CAD build for the part. Positions are in the model's coordinates, mm. Face numbers are marked on the shaded views. A direction names the side the tool comes from. Round coordinates to 2 decimals unless told otherwise and drop trailing zeros. Order: outer loops, then holes, each group sorted by start corner. A loop starts at its lowest first (then second) coordinate and runs counter-clockwise, first axis right, second up. Notation, with made-up numbers: M 35,63.25 L 80,63.25 A26 ccw 80,88.25 Z; hole C 30.25,15 d1. An arc over 180 degrees is marked long. Put each result on its own line as item: value.
```python
from build123d import *

# Parameters (mm, degrees)
SKETCH1_W                    = 52.6
SKETCH1_H                    = 21
BASE_FLANGE1_DEPTH           = 2
EDGE_FLANGE1_STRIP_W         = 9
EDGE_FLANGE1_STRIP_H         = 2
EDGE_FLANGE1_STRIP_CUT_DEPTH = 21
EDGE_FLANGE1_DEPTH           = 21
EDGE_FLANGE2_STRIP_W         = 9
EDGE_FLANGE2_STRIP_H         = 2
EDGE_FLANGE2_STRIP_CUT_DEPTH = 21
EDGE_FLANGE2_DEPTH           = 21
EDGE_FLANGE3_STRIP_W         = 9
EDGE_FLANGE3_STRIP_H         = 2
EDGE_FLANGE3_STRIP_CUT_DEPTH = 21
EDGE_FLANGE3_DEPTH           = 21
SKETCH15_W                   = 3.4
SKETCH15_H                   = 7
CUT_EXTRUDE1_DEPTH           = 10
SKETCH16_R                   = 1.25
CUT_EXTRUDE2_DEPTH           = 2
SKETCH18_W                   = 5.7
SKETCH18_H                   = 7
CUT_EXTRUDE3_DEPTH           = 39.376425055
SKETCH19_R                   = 2.95
CUT_EXTRUDE4_DEPTH           = 2
SKETCH20_R                   = 1.25
CUT_EXTRUDE5_DEPTH           = 2
SKETCH21_R                   = 8.25
CUT_EXTRUDE6_DEPTH           = 2
MOVE_FACE1_BY                = 0.8


# Sheet-metal steps are written as plain solids
with BuildPart() as part:
    # Sketch1 → Base-Flange1 (new body)
    with BuildSketch(Plane(origin=(0, 0, 0), x_dir=(1, 0, 0), z_dir=(0, 1, 0))):
        Rectangle(SKETCH1_W, SKETCH1_H)
    extrude(amount=-BASE_FLANGE1_DEPTH)

    # Edge-Flange1 strip (across the edge) → Edge-Flange1 strip cut (cut)
    with BuildSketch(Plane(origin=(-26.3, 0, -10.5), x_dir=(1, 0, 0), z_dir=(0, 0, 1))):
        with Locations((-2, -1)):
            Rectangle(EDGE_FLANGE1_STRIP_W, EDGE_FLANGE1_STRIP_H)
    extrude(amount=EDGE_FLANGE1_STRIP_CUT_DEPTH, mode=Mode.SUBTRACT)

    # Edge-Flange1 section (across the edge) → Edge-Flange1 (add)
    with BuildSketch(Plane(origin=(-26.3, 0, -10.5), x_dir=(1, 0, 0), z_dir=(0, 0, 1))):
        with BuildLine():
            Line((0, 0.5), (0, 23.9))
            Line((0, 23.9), (2, 23.9))
            Line((2, 23.9), (2, 0.5))
            ThreePointArc((2, 0.5), (2.146446609, 0.146446609), (2.5, 0))
            Line((2.5, 0), (2.5, -2))
            ThreePointArc((2.5, -2), (0.732233047, -1.267766953), (0, 0.5))
        make_face()
    extrude(amount=EDGE_FLANGE1_DEPTH)

    # Edge-Flange2 strip (across the edge) → Edge-Flange2 strip cut (cut)
    with BuildSketch(Plane(origin=(-24.3, 23.9, -10.5), x_dir=(0, -1, 0), z_dir=(0, 0, 1))):
        with Locations((-2, -1)):
            Rectangle(EDGE_FLANGE2_STRIP_W, EDGE_FLANGE2_STRIP_H)
    extrude(amount=EDGE_FLANGE2_STRIP_CUT_DEPTH, mode=Mode.SUBTRACT)

    # Edge-Flange2 section (across the edge) → Edge-Flange2 (add)
    with BuildSketch(Plane(origin=(-24.3, 23.9, -10.5), x_dir=(0, -1, 0), z_dir=(0, 0, 1))):
        with BuildLine():
            Line((0, 0.5), (0, 34.8))
            Line((0, 34.8), (2, 34.8))
            Line((2, 34.8), (2, 0.5))
            ThreePointArc((2, 0.5), (2.146446609, 0.146446609), (2.5, 0))
            Line((2.5, 0), (2.5, -2))
            ThreePointArc((2.5, -2), (0.732233047, -1.267766953), (0, 0.5))
        make_face()
    extrude(amount=EDGE_FLANGE2_DEPTH)

    # Edge-Flange3 strip (across the edge) → Edge-Flange3 strip cut (cut)
    with BuildSketch(Plane(origin=(26.3, 0, 10.5), x_dir=(-1, 0, 0), z_dir=(0, 0, -1))):
        with Locations((-2, -1)):
            Rectangle(EDGE_FLANGE3_STRIP_W, EDGE_FLANGE3_STRIP_H)
    extrude(amount=EDGE_FLANGE3_STRIP_CUT_DEPTH, mode=Mode.SUBTRACT)

    # Edge-Flange3 section (across the edge) → Edge-Flange3 (add)
    with BuildSketch(Plane(origin=(26.3, 0, 10.5), x_dir=(-1, 0, 0), z_dir=(0, 0, -1))):
        with BuildLine():
            Line((0, 0.5), (0, 21.6))
            Line((0, 21.6), (2, 21.6))
            Line((2, 21.6), (2, 0.5))
            ThreePointArc((2, 0.5), (2.146446609, 0.146446609), (2.5, 0))
            Line((2.5, 0), (2.5, -2))
            ThreePointArc((2.5, -2), (0.732233047, -1.267766953), (0, 0.5))
        make_face()
    extrude(amount=EDGE_FLANGE3_DEPTH)

    # Sketch15 → Cut-Extrude1 (cut)
    with BuildSketch(Plane(origin=(0, 23.9, 0), x_dir=(1, 0, 0), z_dir=(0, 1, 0))):
        with Locations((8.8, 0)):
            Rectangle(SKETCH15_W, SKETCH15_H)
    extrude(amount=-CUT_EXTRUDE1_DEPTH, mode=Mode.SUBTRACT)

    # Sketch16 → Cut-Extrude2 (cut)
    with BuildSketch(Plane(origin=(0, 23.9, 0), x_dir=(1, 0, 0), z_dir=(0, 1, 0))):
        with Locations(Location((4.1, 7.8, 0), (0, 0, 180))):
            Circle(SKETCH16_R)
        with Locations(Location((-15.9, -7.3, 0), (0, 0, 180))):
            Circle(SKETCH16_R)
    extrude(amount=-CUT_EXTRUDE2_DEPTH, mode=Mode.SUBTRACT)

    # Sketch18 → Cut-Extrude3 (cut, through all)
    with BuildSketch(Plane(origin=(0, 23.9, 0), x_dir=(1, 0, 0), z_dir=(0, 1, 0))):
        with Locations((9.95, 0)):
            Rectangle(SKETCH18_W, SKETCH18_H)
    extrude(amount=-CUT_EXTRUDE3_DEPTH, mode=Mode.SUBTRACT)

    # Sketch19 → Cut-Extrude4 (cut)
    with BuildSketch(Plane.ZY.offset(26.3)):
        with Locations(Location((0, 10.95, 0), (0, 0, 270))):
            Circle(SKETCH19_R)
    extrude(amount=-CUT_EXTRUDE4_DEPTH, mode=Mode.SUBTRACT)

    # Sketch20 → Cut-Extrude5 (cut)
    with BuildSketch(Plane.XZ.offset(2)):
        with Locations(Location((-16.55, 7.1, 0), (0, 0, 270))):
            Circle(SKETCH20_R)
        with Locations(Location((3.05, 7.1, 0), (0, 0, 270))):
            Circle(SKETCH20_R)
        with Locations(Location((18.05, 7.1, 0), (0, 0, 270))):
            Circle(SKETCH20_R)
        with Locations(Location((-16.55, -7.1, 0), (0, 0, 270))):
            Circle(SKETCH20_R)
        with Locations(Location((3.05, -7.1, 0), (0, 0, 270))):
            Circle(SKETCH20_R)
        with Locations(Location((18.05, -7.1, 0), (0, 0, 270))):
            Circle(SKETCH20_R)
    extrude(amount=-CUT_EXTRUDE5_DEPTH, mode=Mode.SUBTRACT)

    # Sketch21 → Cut-Extrude6 (cut)
    with BuildSketch(Plane(origin=(26.3, 0, 0), x_dir=(0, 0, -1), z_dir=(1, 0, 0))):
        with Locations(Location((0, 10.95, 0), (0, 0, 90))):
            Circle(SKETCH21_R)
    extrude(amount=-CUT_EXTRUDE6_DEPTH, mode=Mode.SUBTRACT)

    # Move Face1: a face moved outward by 0.8
    extrude(part.faces().sort_by_distance((25.3, 21.6, 0))[0], amount=MOVE_FACE1_BY, dir=(0, 1, 0))


solid = part.part
```
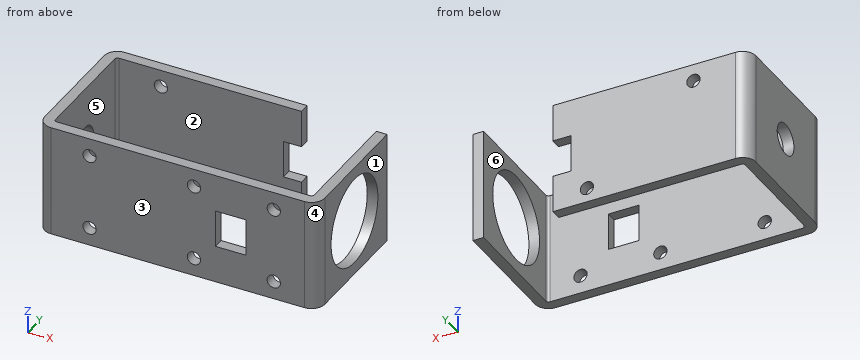
Item 1: Pin check, flat tips, straight feed: P1, Ø1, axis at y = -1, z = -1, coming from the -X side; P2, Ø0.6, axis at y = 23, z = 8, coming from the +X side. Stop position of each tip, or through.
Answers below:
P1: x = -26.09
P2: x = 10.5
Item 2: Mould opens along X. For the marked faces 1, 2 and 3 say: pulls with the +X half, pulls with the -X half, needs draft (parallel to the pull), parting line crosses it, or undercut.
Answers below:
face 1: pulls with the +X half
face 2: undercut
face 3: needs draft
Item 3: Probe line 1 along X through (y, z) = (20, 2); line 2 along X through (y, z) = (22, -8); line 3 along Y through (x, z) = (3.5, -2.5). List the from-to ranges inside material, lowest first. Write a range as [from, to].
Answers below:
line 1: [-26.3, -24.3], [24.3, 26.3]
line 2: [-26.23, 2.87], [5.33, 10.5], [24.3, 26.3]
line 3: [-2, 0], [21.9, 23.9]
Item 4: Band-saw the part on B-B on z = 1.5. Give the cut face in (x, y), and give its area (3 significant figures).
Answers below:
outline: M -26.3,0.5 A2.5 ccw -23.8,-2 L 7.1,-2 L 7.1,0 L -23.8,0 A0.5 cw -24.3,0.5 L -24.3,8.41 L -26.3,8.41 Z; M -26.3,13.49 L -24.3,13.49 L -24.3,21.4 A0.5 cw -23.8,21.9 L 7.1,21.9 L 7.1,23.9 L -23.8,23.9 A2.5 ccw -26.3,21.4 Z; M 12.8,-2 L 23.8,-2 A2.5 ccw 26.3,0.5 L 26.3,2.84 L 24.3,2.84 L 24.3,0.5 A0.5 cw 23.8,0 L 12.8,0 Z; M 24.3,19.06 L 26.3,19.06 L 26.3,22.4 L 24.3,22.4 Z
area: 203 mm²
Item 5: Band-saw the part on D-D on x = -15.9. Give the cut face in (y, z).
Answers below:
outline: M -2,-10.5 L 0,-10.5 L 0,-8.17 L -2,-8.17 Z; M -2,-6.03 L 0,-6.03 L 0,6.03 L -2,6.03 Z; M -2,8.17 L 0,8.17 L 0,10.5 L -2,10.5 Z; M 21.9,-10.5 L 23.9,-10.5 L 23.9,6.05 L 21.9,6.05 Z; M 21.9,8.55 L 23.9,8.55 L 23.9,10.5 L 21.9,10.5 Z
Item 6: Band-saw the part on C-C on y = 10.95. Give the cut face in (x, z), and give its area (3 significant figures).
Answers below:
outline: M -26.3,-10.5 L -24.3,-10.5 L -24.3,-2.95 L -26.3,-2.95 Z; M -26.3,2.95 L -24.3,2.95 L -24.3,10.5 L -26.3,10.5 Z; M 24.3,-10.5 L 26.3,-10.5 L 26.3,-8.25 L 24.3,-8.25 Z; M 24.3,8.25 L 26.3,8.25 L 26.3,10.5 L 24.3,10.5 Z
area: 39.2 mm²
Item 7: Band-saw the part on A-A on x = -4. Give the cut face in (y, z).
Answers below:
outline: M -2,-10.5 L 0,-10.5 L 0,10.5 L -2,10.5 Z; M 21.9,-10.5 L 23.9,-10.5 L 23.9,10.5 L 21.9,10.5 Z
Item 8: Tool access for the marked faces 4, 5 and 6: list every direction of +Z, -Z, +X, -X, +Y, -Y with a clear straight run to the whole face (end or side of a thin tool).
Answers below:
face 4: +Z, -Z, +X, -Y
face 5: +Z, -Z
face 6: +Z, -Z, +Y
